from build123d import *

# Parameters (mm, degrees)
SKETCH1_R           = 38.3
BOSS_EXTRUDE1_DEPTH = 34.7
SKETCH2_R           = 2.6
CUT_EXTRUDE2_DEPTH  = 34.7
SKETCH4_R           = 5.6
CUT_EXTRUDE3_DEPTH  = 3.7
CUT_EXTRUDE4_START  = -3.7
SKETCH5_R           = 5.6
CUT_EXTRUDE4_DEPTH  = 3.7
SKETCH6_R           = 1.65
CUT_EXTRUDE5_DEPTH  = 65.326277679


with BuildPart() as part:
    # Sketch1 → Boss-Extrude1 (new body)
    with BuildSketch(Plane(origin=(0, 0, 0), x_dir=(1, 0, 0), z_dir=(0, 1, 0))):
        with Locations(Location((0, 0, 0), (0, 0, 270))):
            Circle(SKETCH1_R)
    extrude(amount=BOSS_EXTRUDE1_DEPTH)

    # Sketch2 → Cut-Extrude2 (cut)
    with BuildSketch(Plane.XZ):
        with Locations(Location((0, 0, 0), (0, 0, 270))):
            Circle(SKETCH2_R)
    extrude(amount=-CUT_EXTRUDE2_DEPTH, mode=Mode.SUBTRACT)

    # Sketch4 → Cut-Extrude3 (cut)
    with BuildSketch(Plane.XZ):
        with Locations(Location((0, 0, 0), (0, 0, 270))):
            Circle(SKETCH4_R)
    extrude(amount=-CUT_EXTRUDE3_DEPTH, mode=Mode.SUBTRACT)

    # Sketch5 → Cut-Extrude4 (cut)
    with BuildSketch(Plane(origin=(0, 34.7, 0), x_dir=(1, 0, 0), z_dir=(0, 1, 0)).offset(CUT_EXTRUDE4_START)):
        with Locations(Location((0, 0, 0), (0, 0, 90))):
            Circle(SKETCH5_R)
    extrude(amount=CUT_EXTRUDE4_DEPTH, mode=Mode.SUBTRACT)

    # Sketch6 → Cut-Extrude5 (cut, through all)
    with BuildSketch(Plane(origin=(0, 34.7, 0), x_dir=(1, 0, 0), z_dir=(0, 1, 0))):
        with Locations(Location((0, 11.5, 0), (0, 0, 270))):
            Circle(SKETCH6_R)
        with Locations(Location((11.5, 0, 0), (0, 0, 270))):
            Circle(SKETCH6_R)
        with Locations(Location((0, -11.5, 0), (0, 0, 270))):
            Circle(SKETCH6_R)
        with Locations(Location((-11.5, 0, 0), (0, 0, 270))):
            Circle(SKETCH6_R)
    extrude(amount=-CUT_EXTRUDE5_DEPTH, mode=Mode.SUBTRACT)


solid = part.part
For this review, take the finished solid that the model builds, in its own axes (mm). A direction names the side the tool comes from. Give positions to 0.01 mm unless a question says otherwise; leave off trailing zeros. Order: outer loops, then holes, each group sorted by start corner. A loop starts at its lowest first (then second) coordinate and runs counter-clockwise, first axis right, second up. Notation, with made-up numbers: M 62.5,81 L 84.5,81 A17 cw 84.5,107 Z; hole C 50,-8 d6. An arc over 180 degrees is marked long. Answer in a Markdown table with one row per item. Add a question column.
(1) Wall thickness on probe 1 along X at (y, z) = (22.5, 0); probe 2 along X at (y, z) = (33.75, 0); probe 3 along X at (y, z) = (19, -11.5): over which ranges is each line inside the solid? List them lowest first. Write a range as [from, to].
(2) Consider section C-C on y = 11. State the section outline as (x, z) points, and give its area (3 significant figures).
(3) Consider section D-D on z = -11.5. State the section outline as (x, y) points.
(4) For faces 1 (the face through (-1, 3.7, 3)), 2 (the face through (-0.246, 32.824, 5.595)), 3 (the face through (-13.1, 17.6, -0.4)), list the 3-axis set-ups (+Z, -Z, +X, -X, +Y, -Y) from which the entire face can be reached by the end or side of a thin tool; tool diameter is ignored.
(5) Consider section A-A on z = 0. State the section outline as (x, y) points.
(6) Consider section B-B on x = 0. State the section outline as (y, z) points, and give its area (3 significant figures).
(7) For pin 1 (6 mm diameter, centred on x = 0, z = 0, fed in from +Y); pin 2 (9 mm diameter, centred on x = 2, z = 2.5, fed in from +Y); pin 3 (6.5 mm diameter, centred on x = 0, z = 0, fed in from -Y); pin 4 (12 mm diameter, centred on y = 12, z = 10.5, fed in from +X), all flat-tipped, find the tip position at first contact; note any pin that passes through.
(8) Mouldability with a two-part tool opening along Z and no side actions: class faces 4 (the face through (11.504, 17.107, 36.531)), 5 (the face through (-8, 34.7, -1)), 6 (the face through (0.78, 17.16, -2.48)) as +Z half, -Z half, draft (parallel to the pull), parting line (faces both ways), or undercut.
Evaluation:
| question | item | result |
|---|---|---|
| 1 | probe 1 | x = [-38.3, -13.15], [-9.85, -2.6], [2.6, 9.85], [13.15, 38.3] |
| 1 | probe 2 | x = [-38.3, -13.15], [-9.85, -5.6], [5.6, 9.85], [13.15, 38.3] |
| 1 | probe 3 | x = [-36.53, -1.65], [1.65, 36.53] |
| 2 | outline | C 0,0 d76.6; hole C -11.5,0 d3.3; hole C 0,0 d5.2; hole C 0,-11.5 d3.3; hole C 0,11.5 d3.3; hole C 11.5,0 d3.3 |
| 2 | area | 4,550 mm^2 |
| 3 | outline | M -36.53,0 L -1.65,0 L -1.65,34.7 L -36.53,34.7 Z; M 1.65,0 L 36.53,0 L 36.53,34.7 L 1.65,34.7 Z |
| 4 | face 1 | -Y |
| 4 | face 2 | +Y |
| 4 | face 3 | +Y, -Y |
| 5 | outline | M -38.3,0 L -13.15,0 L -13.15,34.7 L -38.3,34.7 Z; M -9.85,0 L -5.6,0 L -5.6,3.7 L -2.6,3.7 L -2.6,31 L -5.6,31 L -5.6,34.7 L -9.85,34.7 Z; M 2.6,3.7 L 5.6,3.7 L 5.6,0 L 9.85,0 L 9.85,34.7 L 5.6,34.7 L 5.6,31 L 2.6,31 Z; M 13.15,0 L 38.3,0 L 38.3,34.7 L 13.15,34.7 Z |
| 6 | outline | M 0,-38.3 L 34.7,-38.3 L 34.7,-13.15 L 0,-13.15 Z; M 0,-9.85 L 34.7,-9.85 L 34.7,-5.6 L 31,-5.6 L 31,-2.6 L 3.7,-2.6 L 3.7,-5.6 L 0,-5.6 Z; M 0,5.6 L 3.7,5.6 L 3.7,2.6 L 31,2.6 L 31,5.6 L 34.7,5.6 L 34.7,9.85 L 0,9.85 Z; M 0,13.15 L 34.7,13.15 L 34.7,38.3 L 0,38.3 Z |
| 6 | area | 2,200 mm^2 |
| 7 | pin 1 | stops at y = 31 |
| 7 | pin 2 | stops at y = 34.7 |
| 7 | pin 3 | stops at y = 3.7 |
| 7 | pin 4 | stops at x = 38.03 |
| 8 | face 4 | parting line |
| 8 | face 5 | draft |
| 8 | face 6 | undercut |
